Could you check a few things on this model? Use its own coordinates, in mm. Face numbers are marked on the shaded views. Round coordinates to 2 decimals unless told otherwise and drop trailing zeros. Loops run counter-clockwise (first coordinate to the right, second up) from the corner with the lowest first, then second, coordinate; pieces in that order, holes last. Notation, with made-up numbers: M 73,-39.75 L 112,-39.75 A17 cw 112,-34.75 Z; hole C 88,19.5 d4. An arc over 180 degrees is marked long. One line per item, written item: value. Start each with the question number.
Q1. Please list where these lines run through material, in increasing order: line 1 along Y through (x, z) = (0, 7); line 2 along Y through (x, z) = (0, 29.9); line 3 along Z through (x, y) = (-2.5, 2).
Q2. Imagine slicing it at C-C (z = 11). Please give me the cut outline in (x, y).
Q3. Imagine slicing it at A-A (y = 0). Please give me the cut outline in (x, z).
Q4. Imagine slicing it at D-D (z = 29.5). Please give me the cut outline in (x, y).
Q5. Thinking about a two-plate mould opening in X: for the marked faces 1 and 2, which applies, released by +X, released by -X, zero draft, split by the parting line, or undercut?
Q6. I'm going to push flat-ended pins straight in: pin 1 Ø4 at (y, z) = (-2.5, 21.5) entering from -X; pin 2 Ø1.5 at (x, y) = (-0.5, 0) entering from -Z; pin 3 Ø1 at (x, z) = (1.5, 10) entering from +Y. Where does each tip first touch, or does it pass through?
from build123d import *

# Parameters (mm, degrees)
F0_R     = 3.7338
F1_DEPTH = 27.8003
F2_R     = 2.2606
F3_DEPTH = 4.1021
F4_R     = 1.0414
F5_DEPTH = 47.0154
F6_R     = 2.53873
F7_DEPTH = 26.9494
F8_R     = 3.7338
F9_DEPTH = 26.3144


with BuildPart() as f1:
    # F0 (on Top) → F1 (new body)
    with BuildSketch(Plane.XY):
        Circle(F0_R)
    extrude(amount=F1_DEPTH)

    # F2 (on face) → F3 (join)
    with BuildSketch(Plane.XY.offset(27.8003)):
        Circle(F2_R)
    extrude(amount=F3_DEPTH)

    # F4 (on face) → F5 (cut)
    with BuildSketch(Plane.XY.offset(31.9024)):
        Circle(F4_R)
    extrude(amount=-F5_DEPTH, mode=Mode.SUBTRACT)

    # F6 (on face) → F7 (cut)
    with BuildSketch(Plane(origin=(0, 0, 0), x_dir=(1, 0, 0), z_dir=(0, 0, -1))):
        Circle(F6_R)
    extrude(amount=-F7_DEPTH, mode=Mode.SUBTRACT)

    # F8 (on face) → F9 (join)
    with BuildSketch(Plane(origin=(0, 0, 0), x_dir=(1, 0, 0), z_dir=(0, 0, -1))):
        Circle(F8_R)
        with BuildLine():
            Line((1.1798710111, 2.2479), (2.2479, 2.2479))
            Line((2.2479, 2.2479), (2.2479, 1.1798710111))
            ThreePointArc((2.2479, 1.1798710111), (2.4649504234, 0.6075931393), (2.53873, 0))
            ThreePointArc((2.53873, 0), (2.4649504234, -0.6075931393), (2.2479, -1.1798710111))
            Line((2.2479, -1.1798710111), (2.2479, -2.2479))
            Line((2.2479, -2.2479), (1.1798710111, -2.2479))
            ThreePointArc((1.1798710111, -2.2479), (0, -2.53873), (-1.1798710111, -2.2479))
            Line((-1.1798710111, -2.2479), (-2.2479, -2.2479))
            Line((-2.2479, -2.2479), (-2.2479, -1.1798710111))
            ThreePointArc((-2.2479, -1.1798710111), (-2.53873, 0), (-2.2479, 1.1798710111))
            Line((-2.2479, 1.1798710111), (-2.2479, 2.2479))
            Line((-2.2479, 2.2479), (-1.1798710111, 2.2479))
            ThreePointArc((-1.1798710111, 2.2479), (0, 2.53873), (1.1798710111, 2.2479))
        make_face(mode=Mode.SUBTRACT)
        with BuildLine():
            Line((-1.1798710111, 2.2479), (1.1798710111, 2.2479))
            ThreePointArc((1.1798710111, 2.2479), (0, 2.53873), (-1.1798710111, 2.2479))
        make_face()
        with BuildLine():
            ThreePointArc((2.53873, 0), (2.4649504234, 0.6075931393), (2.2479, 1.1798710111))
            Line((2.2479, 1.1798710111), (2.2479, -1.1798710111))
            ThreePointArc((2.2479, -1.1798710111), (2.4649504234, -0.6075931393), (2.53873, 0))
        make_face()
        with BuildLine():
            Line((-2.2479, -1.1798710111), (-2.2479, 1.1798710111))
            ThreePointArc((-2.2479, 1.1798710111), (-2.53873, 0), (-2.2479, -1.1798710111))
        make_face()
        with BuildLine():
            ThreePointArc((-1.1798710111, -2.2479), (0, -2.53873), (1.1798710111, -2.2479))
            Line((1.1798710111, -2.2479), (-1.1798710111, -2.2479))
        make_face()
    extrude(amount=-F9_DEPTH)


solid = f1.part
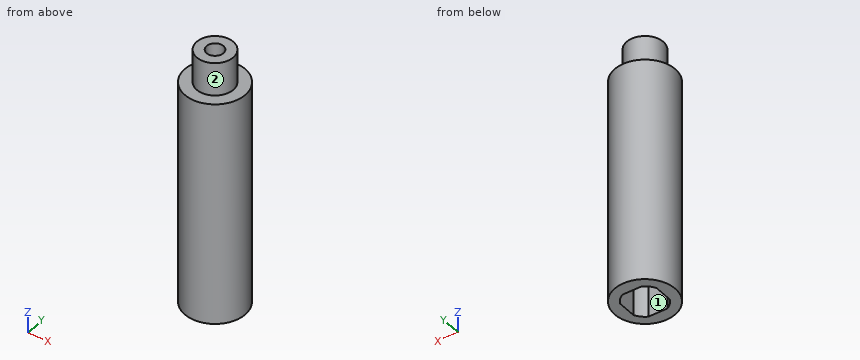
Report:
1. line 1: y = -3.73 to -2.25, 2.25 to 3.73
1. line 2: y = -2.26 to -1.04, 1.04 to 2.26
1. line 3: z = 0 to 27.8
2. outline: C 0,0 d7.47; hole M -2.25,-1.18 A2.54 ccw -1.18,-2.25 L 1.18,-2.25 A2.54 ccw 2.25,-1.18 L 2.25,1.18 A2.54 ccw 1.18,2.25 L -1.18,2.25 A2.54 ccw -2.25,1.18 Z
3. outline: M -3.73,0 L -2.25,0 L -2.25,26.31 L -2.54,26.31 L -2.54,26.95 L -1.04,26.95 L -1.04,31.9 L -2.26,31.9 L -2.26,27.8 L -3.73,27.8 Z; M 1.04,26.95 L 2.54,26.95 L 2.54,26.31 L 2.25,26.31 L 2.25,0 L 3.73,0 L 3.73,27.8 L 2.26,27.8 L 2.26,31.9 L 1.04,31.9 Z
4. outline: C 0,0 d4.52; hole C 0,0 d2.08
5. face 1: undercut
5. face 2: split by the parting line
6. pin 1: stops at x = -3.7
6. pin 2: stops at z = 26.95
6. pin 3: stops at y = 3.6
